```python
from build123d import *
from build123d.topology import SkipClean

# Parameters (mm, degrees)
SKETCH1_R           = 5
BOSS_EXTRUDE1_DEPTH = 10
BOSS_EXTRUDE2_DEPTH = 50


with BuildPart() as part:
    # Sketch1 → Boss-Extrude1 (new body)
    with BuildSketch(Plane.XY):
        with BuildLine():
            Line((-5, 48.660254038), (-10, 40))
            Line((-10, 40), (-10.868896713, 38.495026747))
            ThreePointArc((-10.868896713, 38.495026747), (-20, 34.641016151), (-27.903222726, 28.660254038))
            Line((-27.903222726, 28.660254038), (-29.641016151, 28.660254038))
            Line((-29.641016151, 28.660254038), (-39.641016151, 28.660254038))
            Line((-39.641016151, 28.660254038), (-44.641016151, 20))
            Line((-44.641016151, 20), (-39.641016151, 11.339745962))
            Line((-39.641016151, 11.339745962), (-38.772119439, 9.834772709))
            ThreePointArc((-38.772119439, 9.834772709), (-40, 0), (-38.772119439, -9.834772709))
            Line((-38.772119439, -9.834772709), (-39.641016151, -11.339745962))
            Line((-39.641016151, -11.339745962), (-44.641016151, -20))
            Line((-44.641016151, -20), (-39.641016151, -28.660254038))
            Line((-39.641016151, -28.660254038), (-29.641016151, -28.660254038))
            Line((-29.641016151, -28.660254038), (-27.903222726, -28.660254038))
            ThreePointArc((-27.903222726, -28.660254038), (-20, -34.641016151), (-10.868896713, -38.495026747))
            Line((-10.868896713, -38.495026747), (-10, -40))
            Line((-10, -40), (-5, -48.660254038))
            Line((-5, -48.660254038), (5, -48.660254038))
            Line((5, -48.660254038), (10, -40))
            Line((10, -40), (10.868896713, -38.495026747))
            ThreePointArc((10.868896713, -38.495026747), (20, -34.641016151), (27.903222726, -28.660254038))
            Line((27.903222726, -28.660254038), (29.641016151, -28.660254038))
            Line((29.641016151, -28.660254038), (39.641016151, -28.660254038))
            Line((39.641016151, -28.660254038), (44.641016151, -20))
            Line((44.641016151, -20), (39.641016151, -11.339745962))
            Line((39.641016151, -11.339745962), (38.772119439, -9.834772709))
            ThreePointArc((38.772119439, -9.834772709), (40, 0), (38.772119439, 9.834772709))
            Line((38.772119439, 9.834772709), (39.641016151, 11.339745962))
            Line((39.641016151, 11.339745962), (44.641016151, 20))
            Line((44.641016151, 20), (39.641016151, 28.660254038))
            Line((39.641016151, 28.660254038), (29.641016151, 28.660254038))
            Line((29.641016151, 28.660254038), (27.903222726, 28.660254038))
            ThreePointArc((27.903222726, 28.660254038), (20, 34.641016151), (10.868896713, 38.495026747))
            Line((10.868896713, 38.495026747), (10, 40))
            Line((10, 40), (5, 48.660254038))
            Line((5, 48.660254038), (-5, 48.660254038))
        make_face()
        Circle(SKETCH1_R, mode=Mode.SUBTRACT)
        with BuildLine():
            Line((-2.5, 9.682458366), (-2.5, 34.910600109))
            ThreePointArc((-2.5, 34.910600109), (-17.5, 30.310889132), (-28.983466556, 19.620363564))
            Line((-28.983466556, 19.620363564), (-7.135254916, 7.006292692))
            ThreePointArc((-7.135254916, 7.006292692), (-5, 8.660254038), (-2.5, 9.682458366))
        make_face(mode=Mode.SUBTRACT)
        with BuildLine():
            Line((2.5, 34.910600109), (2.5, 9.682458366))
            ThreePointArc((2.5, 9.682458366), (5, 8.660254038), (7.135254916, 7.006292692))
            Line((7.135254916, 7.006292692), (28.983466556, 19.620363564))
            ThreePointArc((28.983466556, 19.620363564), (17.5, 30.310889132), (2.5, 34.910600109))
        make_face(mode=Mode.SUBTRACT)
        with BuildLine():
            Line((31.483466556, 15.290236545), (9.635254916, 2.676165673))
            ThreePointArc((9.635254916, 2.676165673), (10, 0), (9.635254916, -2.676165673))
            Line((9.635254916, -2.676165673), (31.483466556, -15.290236545))
            ThreePointArc((31.483466556, -15.290236545), (35, 0), (31.483466556, 15.290236545))
        make_face(mode=Mode.SUBTRACT)
        with BuildLine():
            Line((28.983466556, -19.620363564), (7.135254916, -7.006292692))
            ThreePointArc((7.135254916, -7.006292692), (5, -8.660254038), (2.5, -9.682458366))
            Line((2.5, -9.682458366), (2.5, -34.910600109))
            ThreePointArc((2.5, -34.910600109), (17.5, -30.310889132), (28.983466556, -19.620363564))
        make_face(mode=Mode.SUBTRACT)
        with BuildLine():
            Line((-2.5, -34.910600109), (-2.5, -9.682458366))
            ThreePointArc((-2.5, -9.682458366), (-5, -8.660254038), (-7.135254916, -7.006292692))
            Line((-7.135254916, -7.006292692), (-28.983466556, -19.620363564))
            ThreePointArc((-28.983466556, -19.620363564), (-17.5, -30.310889132), (-2.5, -34.910600109))
        make_face(mode=Mode.SUBTRACT)
        with BuildLine():
            Line((-31.483466556, -15.290236545), (-9.635254916, -2.676165673))
            ThreePointArc((-9.635254916, -2.676165673), (-10, 0), (-9.635254916, 2.676165673))
            Line((-9.635254916, 2.676165673), (-31.483466556, 15.290236545))
            ThreePointArc((-31.483466556, 15.290236545), (-35, 0), (-31.483466556, -15.290236545))
        make_face(mode=Mode.SUBTRACT)
    extrude(amount=BOSS_EXTRUDE1_DEPTH)

    # Sketch2 → Boss-Extrude2 (add)
    with SkipClean():  # the faces are left unmerged after this step: merging them gives an invalid solid
        with BuildSketch(Plane.XY.offset(10)):
            with BuildLine():
                Line((-44.641016151, 20), (-38.772119439, 9.834772709))
                ThreePointArc((-38.772119439, 9.834772709), (-40, 0), (-38.772119439, -9.834772709))
                Line((-38.772119439, -9.834772709), (-44.641016151, -20))
                Line((-44.641016151, -20), (-39.641016151, -28.660254038))
                Line((-39.641016151, -28.660254038), (-27.903222726, -28.660254038))
                ThreePointArc((-27.903222726, -28.660254038), (-20, -34.641016151), (-10.868896713, -38.495026747))
                Line((-10.868896713, -38.495026747), (-5, -48.660254038))
                Line((-5, -48.660254038), (5, -48.660254038))
                Line((5, -48.660254038), (10.868896713, -38.495026747))
                ThreePointArc((10.868896713, -38.495026747), (20, -34.641016151), (27.903222726, -28.660254038))
                Line((27.903222726, -28.660254038), (39.641016151, -28.660254038))
                Line((39.641016151, -28.660254038), (44.641016151, -20))
                Line((44.641016151, -20), (38.772119439, -9.834772709))
                ThreePointArc((38.772119439, -9.834772709), (40, 0), (38.772119439, 9.834772709))
                Line((38.772119439, 9.834772709), (44.641016151, 20))
                Line((44.641016151, 20), (39.641016151, 28.660254038))
                Line((39.641016151, 28.660254038), (27.903222726, 28.660254038))
                ThreePointArc((27.903222726, 28.660254038), (20, 34.641016151), (10.868896713, 38.495026747))
                Line((10.868896713, 38.495026747), (5, 48.660254038))
                Line((5, 48.660254038), (-5, 48.660254038))
                Line((-5, 48.660254038), (-10.868896713, 38.495026747))
                ThreePointArc((-10.868896713, 38.495026747), (-20, 34.641016151), (-27.903222726, 28.660254038))
                Line((-27.903222726, 28.660254038), (-39.641016151, 28.660254038))
                Line((-39.641016151, 28.660254038), (-44.641016151, 20))
            make_face()
            with BuildLine():
                ThreePointArc((31.483466556, 15.290236545), (34.109539204, 7.844701095), (35, 0))
                ThreePointArc((35, 0), (34.109539204, -7.844701095), (31.483466556, -15.290236545))
                ThreePointArc((31.483466556, -15.290236545), (30.310889132, -17.5), (28.983466556, -19.620363564))
                ThreePointArc((28.983466556, -19.620363564), (17.5, -30.310889132), (2.5, -34.910600109))
                ThreePointArc((2.5, -34.910600109), (0, -35), (-2.5, -34.910600109))
                ThreePointArc((-2.5, -34.910600109), (-17.5, -30.310889132), (-28.983466556, -19.620363564))
                ThreePointArc((-28.983466556, -19.620363564), (-30.310889132, -17.5), (-31.483466556, -15.290236545))
                ThreePointArc((-31.483466556, -15.290236545), (-35, 0), (-31.483466556, 15.290236545))
                ThreePointArc((-31.483466556, 15.290236545), (-30.310889132, 17.5), (-28.983466556, 19.620363564))
                ThreePointArc((-28.983466556, 19.620363564), (-17.5, 30.310889132), (-2.5, 34.910600109))
                ThreePointArc((-2.5, 34.910600109), (0, 35), (2.5, 34.910600109))
                ThreePointArc((2.5, 34.910600109), (17.5, 30.310889132), (28.983466556, 19.620363564))
                ThreePointArc((28.983466556, 19.620363564), (30.310889132, 17.5), (31.483466556, 15.290236545))
            make_face(mode=Mode.SUBTRACT)
        extrude(amount=BOSS_EXTRUDE2_DEPTH)


solid = part.part
```
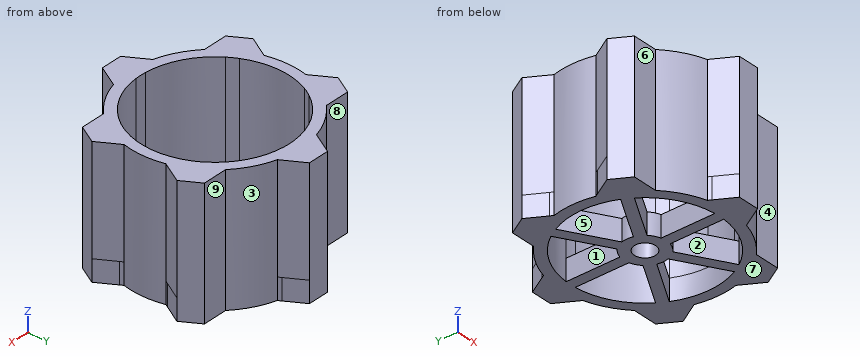
For this review, take the finished solid that the model builds, in its own axes (mm). Face numbers are marked on the shaded views. A direction names the side the tool comes from. Coordinates: 2 decimals unless noted, no trailing zeros. Loops run counter-clockwise (first coordinate to the right, second up) from the corner with the lowest first, then second, coordinate; pieces in that order, holes last. Notation, with made-up numbers: (-26, 85) -> (-3, 85) arc R26 ccw to (-3, 124) -> close; hole circle Ø3 at (-36.75, -16). An arc over 180 degrees is marked (long way). Return JSON: item names as keys, results as strings. Group by question number.
(1) Consider section B-B, the plane x = 19. Give the boundary of the cut face in (y, z), plus the area to 3 significant figures.
(2) Tool access review of the marked faces 5, 6, 7, 8 and 9: name each direction out of +Z, -Z, +X, -X, +Y, -Y from which nothing blocks a thin tool from reaching the whole face with its end or side.
(3) To check wall thickness, follow L1, parallel to Y at x = 0, z = 7.75; L2, parallel to X at y = 29.5, z = 9.5; L3, parallel to Y at x = 23.5, z = 47. State the ranges of each line that lie inside material, in increasing order.
(4) Mouldability with a two-part tool opening along X and no side actions: class the marked faces 1, 2, 3 and 4 as pulls with the +X half, pulls with the -X half, needs draft (parallel to the pull), parting line crosses it, or undercut.
(5) Consider section C-C, the plane z = 6. Count the separate pieces of the cut face and the enclosed holes in it, plus the area to 3 significant figures.
(6) Consider section A-A, the plane x = 0. Give the boundary of the cut face in (y, z), plus the area to 3 significant figures.
(7) Consider section D-D, the plane y = 42. Give the boundary of the cut face in (x, z).
(8) For pin 1 Ø11 at (y, z) = (24, 3) entering from -X; pin 2 Ø8 at (y, z) = (-28.5, 5.5) entering from -X; pin 3 Ø12 at (x, y) = (-12, -10.5) entering from +Z; pin 4 Ø3.5 at (x, z) = (-34.5, 40.5) entering from -Y, all flat-tipped, find the tip position at first contact; note any pin that passes through.
Results below:
{
 "1": {"outline": "(-35.2, 0) -> (-29.39, 0) -> (-29.39, 60) -> (-35.2, 60) -> close; (-13.86, 0) -> (-8.08, 0) -> (-8.08, 10) -> (-13.86, 10) -> close; (8.08, 0) -> (13.86, 0) -> (13.86, 10) -> (8.08, 10) -> close; (29.39, 0) -> (35.2, 0) -> (35.2, 60) -> (29.39, 60) -> close", "area": "812 mm2"},
 "2": {"face 5": "+Z, -Z", "face 6": "+Z, -Z, -X, -Y", "face 7": "-Z, +X, -X, +Y, -Y", "face 8": "+Z, -Z, -X, +Y", "face 9": "+Z, -Z, +X, +Y"},
 "3": {"L1": "y = -48.66 to -5, 5 to 48.66", "L2": "x = -27.01 to -18.83, -2.5 to 2.5, 18.83 to 27.01", "L3": "y = -32.37 to -25.94, 25.94 to 32.37"},
 "4": {"face 1": "undercut", "face 2": "undercut", "face 3": "pulls with the +X half", "face 4": "needs draft"},
 "5": {"separate pieces": "1", "enclosed holes": "7", "area": "3,000 mm2"},
 "6": {"outline": "(-48.66, 0) -> (-5, 0) -> (-5, 10) -> (-35, 10) -> (-35, 60) -> (-48.66, 60) -> close; (5, 0) -> (48.66, 0) -> (48.66, 60) -> (35, 60) -> (35, 10) -> (5, 10) -> close", "area": "2,240 mm2"},
 "7": {"outline": "(-8.85, 0) -> (8.85, 0) -> (8.85, 60) -> (-8.85, 60) -> close"},
 "8": {"pin 1": "stops at x = -44.64", "pin 2": "stops at x = -42.04", "pin 3": "stops at z = 10", "pin 4": "stops at y = -28.66"}
}
